Build history of the part. All positions in model axes, mm. Give positions to 0.01 mm unless a question says otherwise; leave off trailing zeros. Loops run counter-clockwise (first coordinate to the right, second up) from the corner with the lowest first, then second, coordinate; pieces in that order, holes last.
1) Band-saw the part on B-B on z = 1.8. List the corners of the cut face in (x, y), then the cut area to 3 significant figures.
2) Wall check: line 1 (X direction, y = -5, z = 1.4); line 2 (Y direction, x = 25.5, z = 1.4). Give the ranges that are in metal, low to high.
3) Flat gauge pins, fed straight in: P1, Ø0.6, axis at y = -10.5, z = 1.5, coming from the -X side; P2, Ø1, axis at x = -2.5, z = 2, coming from the +Y side. Where does each tip first touch, or does it go through?
4) Band-saw the part on A-A on x = -1. List the corners of the cut face in (y, z).
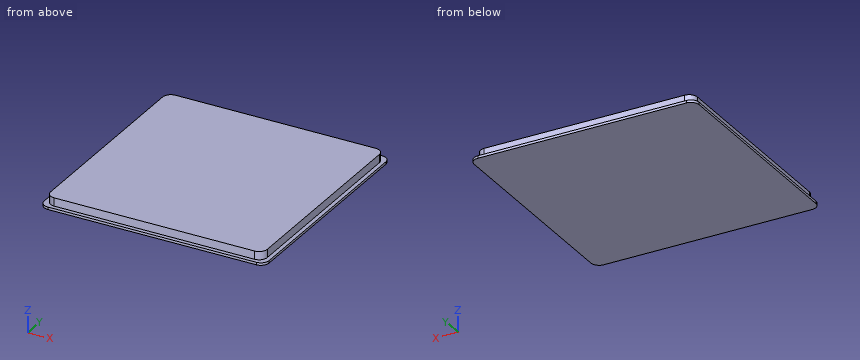
```python
from build123d import *

# Parameters (mm, degrees)
F0_W     = 52.9
F0_H     = 52.9
F1_DEPTH = 2.6
F0_W_2   = 54.9
F0_H_2   = 54.9
F2_DEPTH = 0.6
F3_R     = 2


with BuildPart() as f1:
    # F0 (on Top) → F1 (new body)
    with BuildSketch(Plane.XY):
        Rectangle(F0_W, F0_H)
    extrude(amount=F1_DEPTH)

    # F0 (on Top) → F2 (join)
    with BuildSketch(Plane.XY):
        Rectangle(F0_W_2, F0_H_2)
        Rectangle(F0_W, F0_H, mode=Mode.SUBTRACT)
    extrude(amount=F2_DEPTH)

    # F3
    f3_edges = [f1.edges().sort_by_distance(p)[0] for p in [
        (-26.45, -26.45, 1.6),
        (26.45, -26.45, 1.6),
        (-26.45, 26.45, 1.6),
        (26.45, 26.45, 1.6),
        (-27.45, 27.45, 0.3),
        (-27.45, -27.45, 0.3),
        (27.45, -27.45, 0.3),
        (27.45, 27.45, 0.3),
    ]]
    fillet(f3_edges, radius=F3_R)


solid = f1.part
```
Findings below:
1. outline: (-26.45, -24.45) arc R2 ccw to (-24.45, -26.45) - (24.45, -26.45) arc R2 ccw to (26.45, -24.45) - (26.45, 24.45) arc R2 ccw to (24.45, 26.45) - (-24.45, 26.45) arc R2 ccw to (-26.45, 24.45) - close
1. area: 2,790 mm2
2. line 1: x = -26.45 to 26.45
2. line 2: y = -26.15 to 26.15
3. P1: stops at x = -26.45
3. P2: stops at y = 26.45
4. outline: (-27.45, 0) - (27.45, 0) - (27.45, 0.6) - (26.45, 0.6) - (26.45, 2.6) - (-26.45, 2.6) - (-26.45, 0.6) - (-27.45, 0.6) - close
